Input: dimensioned drawing with shaded views. Units: mm. Origin: part minimum x, y, z. A direction names the side the tool comes from. Give positions to 0.01 mm unless a question says otherwise; leave off trailing zeros. Loops run counter-clockwise (first coordinate to the right, second up) from the corner with the lowest first, then second, coordinate; pieces in that order, holes last.
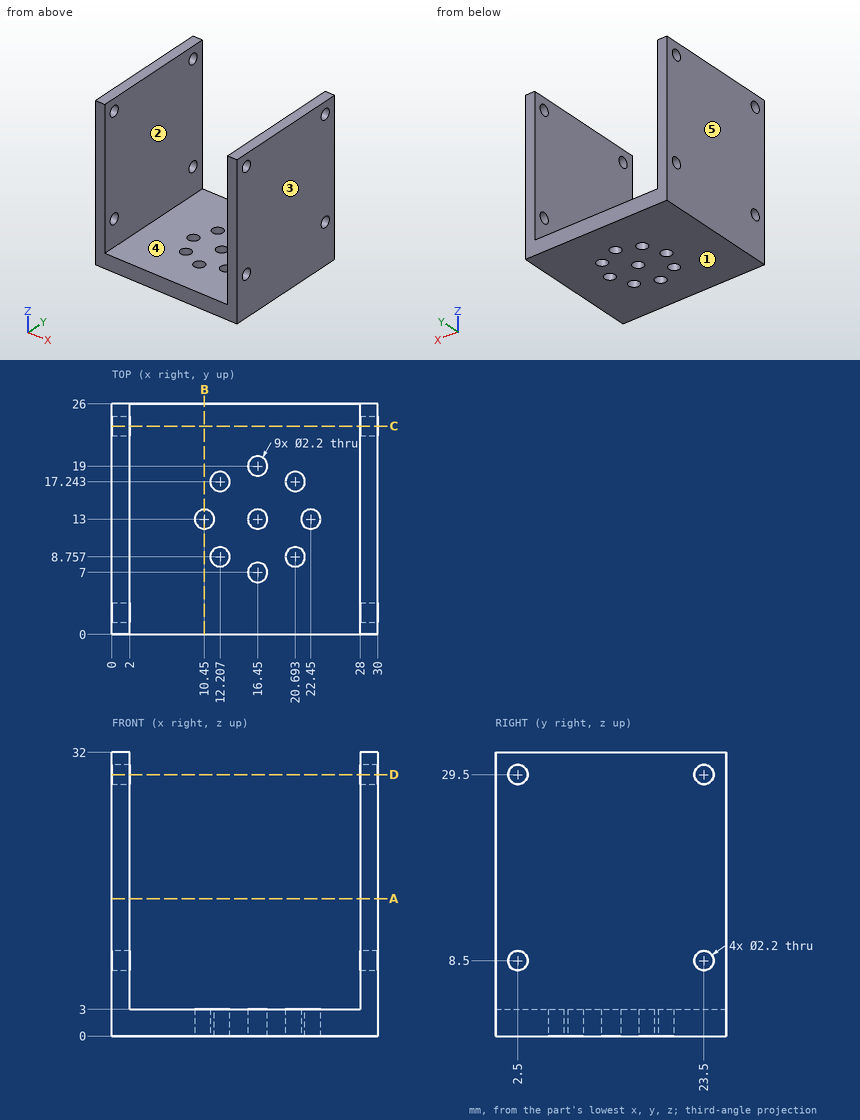
Item 1: Set-up query: the marked faces 4 and 5. Return all of +Z, -Z, +X, -X, +Y, -Y with unobstructed straight access to the full face (end or side cutting, diameter ignored); none if empty.
Values follow:
face 4: +Z, +Y, -Y
face 5: +Z, -Z, -X, +Y, -Y
Item 2: Section query A-A on z = 15.5. Return loops of the section in (x, y).
Values follow:
outline: (0, 0) - (2, 0) - (2, 26) - (0, 26) - close; (28, 0) - (30, 0) - (30, 26) - (28, 26) - close
Item 3: Section query D-D on z = 29.5. Return loops of the section in (x, y).
Values follow:
outline: (0, 0) - (2, 0) - (2, 1.4) - (0, 1.4) - close; (0, 3.6) - (2, 3.6) - (2, 22.4) - (0, 22.4) - close; (0, 24.6) - (2, 24.6) - (2, 26) - (0, 26) - close; (28, 0) - (30, 0) - (30, 1.4) - (28, 1.4) - close; (28, 3.6) - (30, 3.6) - (30, 22.4) - (28, 22.4) - close; (28, 24.6) - (30, 24.6) - (30, 26) - (28, 26) - close
Item 4: Pin query (flat end, axial travel): pin 1 (1.3 mm diameter, centred on x = 10.45, y = 13, fed in from +Z); pin 2 (3.5 mm diameter, centred on x = 12.21, y = 8.76, fed in from +Z). Return the tip coordinate at first contact, or that it passes through.
Values follow:
pin 1: passes through
pin 2: stops at z = 3
Item 5: Draft query along X for the marked faces 1, 2 and 3. Return one class per face: +X half, -X half, draft (parallel to the pull), parting line (faces both ways), or undercut.
Values follow:
face 1: draft
face 2: undercut
face 3: +X half
Item 6: Ray query, probe 1 along Y at (x, z) = (16.45, 2.1); probe 2 along Y at (x, z) = (1.5, 29.5); probe 3 along Z at (x, y) = (29.65, 23.5). Return the intervals inside material, ascending.
Values follow:
probe 1: y = 0 to 5.9, 8.1 to 11.9, 14.1 to 17.9, 20.1 to 26
probe 2: y = 0 to 1.4, 3.6 to 22.4, 24.6 to 26
probe 3: z = 0 to 7.4, 9.6 to 28.4, 30.6 to 32
Item 7: Section query C-C on y = 23.5. Return loops of the section in (x, z).
Values follow:
outline: (0, 0) - (30, 0) - (30, 7.4) - (28, 7.4) - (28, 3) - (2, 3) - (2, 7.4) - (0, 7.4) - close; (0, 9.6) - (2, 9.6) - (2, 28.4) - (0, 28.4) - close; (0, 30.6) - (2, 30.6) - (2, 32) - (0, 32) - close; (28, 9.6) - (30, 9.6) - (30, 28.4) - (28, 28.4) - close; (28, 30.6) - (30, 30.6) - (30, 32) - (28, 32) - close
Item 8: Section query B-B on x = 10.45. Return loops of the section in (y, z), plus the area to 3 significant figures.
Values follow:
outline: (0, 0) - (11.9, 0) - (11.9, 3) - (0, 3) - close; (14.1, 0) - (26, 0) - (26, 3) - (14.1, 3) - close
area: 71.4 mm2
